Work out the finished part from the listing and answer in its coordinate system (mm). A direction names the side the tool comes from. Coordinates: 2 decimals unless noted, no trailing zeros. Order: outer loops, then holes, each group sorted by start corner. A loop starts at its lowest first (then second) coordinate and runs counter-clockwise, first axis right, second up.
1. A flat-ended cylindrical pin translates along its axis: pin 1 Ø6 at (x, y) = (35.78, 18.05) entering from +Z. Find the tip coordinate at first contact, or state that the pin passes through.
2. A tool of negligible diameter and unlimited length cuts with its end or side. For faces 1 (the flat face through (42.649, 18, 3)), 2 (the flat face through (31.777, 16, 3)), from which of +Z, -Z, +X, -X, +Y, -Y can it reach the whole face along a straight path? Write none if from no direction.
3. The part is cut by section C-C, the plane z = 2.55. Count the separate pieces of the cut face and the enclosed holes in it, then the cut area to 3 significant figures.
4. The part is cut by section D-D, the plane y = 17.75. Give the vertices of the cut face in (x, z).
5. Determine the mould class of faces 3 (the flat face through (44, 24.054, 3)), 4 (the cylindrical face through (53.438, 17.364, 2.958)), 5 (the flat face through (55.777, 16, 3)) for opening direction X: +X half, -X half, draft (parallel to the pull), parting line (faces both ways), or undercut.
6. The part is cut by section B-B, the plane x = 51.5. Give the vertices of the cut face in (y, z), then the cut area to 3 significant figures.
7. The part is cut by section A-A, the plane y = 10.5. Give the vertices of the cut face in (x, z).
8. Find the intervals of material crossed by probe 1 along X at (y, z) = (18.25, 0.75); probe 2 along X at (y, z) = (16.75, 2.2); probe 3 along X at (y, z) = (13, 5.7), in increasing order.
```python
from build123d import *

# Parameters (mm, degrees)
MODEL_W                  = 23.99999232
MODEL_H                  = 16.699994656
MODEL_R                  = 1.8
RESSALTO_EXTRUS_O1_DEPTH = 6


with BuildPart() as part:
    # Model → Ressalto-extrusão1 (new body)
    with BuildSketch(Plane.XY):
        with Locations((43.7766695, 15.703554206)):
            Rectangle(MODEL_W, MODEL_H)
        with Locations((35.77667206, 18.053553454)):
            Circle(MODEL_R, mode=Mode.SUBTRACT)
        with Locations((43.861433665, 11.553555534)):
            Circle(MODEL_R, mode=Mode.SUBTRACT)
        with Locations((51.77555053, 18.053553454)):
            Circle(MODEL_R, mode=Mode.SUBTRACT)
        Polygon((42.649145536, 19.728924359), (42.649145536, 16.382506676), (42.669242478, 16.286318247), (42.729533303, 16.197543356), (42.970696603, 16.042234191), (43.332060456, 15.936872625), (43.77304988, 15.901752102), (44.214039305, 15.936872625), (44.575403158, 16.042234191), (44.816566458, 16.197543356), (44.876857283, 16.286318247), (44.896954225, 16.382506676), (44.896954225, 19.728924359), (44.876857283, 19.825112787), (44.816566458, 19.913887678), (44.575403158, 20.069196843), (44.214039305, 20.17455841), (43.77304988, 20.209678932), (43.332060456, 20.17455841), (42.970696603, 20.069196843), (42.729533303, 19.913887678), (42.669242478, 19.825112787), align=None, mode=Mode.SUBTRACT)
    extrude(amount=RESSALTO_EXTRUS_O1_DEPTH)


solid = part.part
```
Geometry says:
1. pin 1: stops at z = 6
2. face 1: +Z, -Z
2. face 2: +Z, -Z, -X, +Y, -Y
3. separate pieces: 1
3. enclosed holes: 4
3. area: 361 mm2
4. outline: (31.78, 0) - (34, 0) - (34, 6) - (31.78, 6) - close; (37.55, 0) - (42.65, 0) - (42.65, 6) - (37.55, 6) - close; (44.9, 0) - (50, 0) - (50, 6) - (44.9, 6) - close; (53.55, 0) - (55.78, 0) - (55.78, 6) - (53.55, 6) - close
5. face 3: draft
5. face 4: undercut
5. face 5: +X half
6. outline: (7.35, 0) - (16.27, 0) - (16.27, 6) - (7.35, 6) - close; (19.83, 0) - (24.05, 0) - (24.05, 6) - (19.83, 6) - close
6. area: 78.9 mm2
7. outline: (31.78, 0) - (42.4, 0) - (42.4, 6) - (31.78, 6) - close; (45.32, 0) - (55.78, 0) - (55.78, 6) - (45.32, 6) - close
8. probe 1: x = 31.78 to 33.99, 37.57 to 42.65, 44.9 to 49.99, 53.56 to 55.78
8. probe 2: x = 31.78 to 34.54, 37.02 to 42.65, 44.9 to 50.53, 53.02 to 55.78
8. probe 3: x = 31.78 to 42.79, 44.93 to 55.78
